Read the model definition and answer for the solid it produces. Units are mm, in the model's axes. Face numbers are marked on the shaded views. A direction names the side the tool comes from. Coordinates: 2 decimals unless noted, no trailing zeros. Loops run counter-clockwise (first coordinate to the right, second up) from the corner with the lowest first, then second, coordinate; pieces in that order, holes last. Notation, with made-up numbers: (-16.5, 14) -> (34.5, 14) arc R20 cw to (34.5, 41) -> close; hole circle Ø3 at (-28.75, 45). An arc over 180 degrees is marked (long way). Answer in a Markdown table with one row per item.
```python
from build123d import *
from build123d.topology import SkipClean

# Parameters (mm, degrees)
SKETCH1_R                    = 10.16
BOSS_EXTRUDE1_DEPTH          = 101.6
SKETCH3_R                    = 12.7
SKETCH3_R_2                  = 3.302
BOSS_EXTRUDE2_DEPTH          = 12.7
SKETCH5_W                    = 50.328091527
SKETCH5_H                    = 177.713548071
CUT_EXTRUDE2_DEPTH           = 122.062113097
SKETCH4_W                    = 0.976
SKETCH4_H                    = 5
CUT_EXTRUDE3_DEPTH           = 11.684
SKETCH4_3_R                  = 3.175
CUT_EXTRUDE4_DEPTH           = 6.35
CUT_EXTRUDE4_DRAFT           = -5
CUT_EXTRUDE4_PROFILE_2_DEPTH = 6.35
CUT_EXTRUDE4_PROFILE_2_DRAFT = -5
CUT_EXTRUDE4_PROFILE_3_DEPTH = 6.35
CUT_EXTRUDE4_PROFILE_3_DRAFT = -5
CUT_EXTRUDE4_PROFILE_4_DEPTH = 6.35
CUT_EXTRUDE4_PROFILE_4_DRAFT = -5
CUT_EXTRUDE5_DEPTH           = 124.013791019


with BuildPart() as part:
    # Sketch1 → Boss-Extrude1 (new body)
    with BuildSketch(Plane.XY):
        Circle(SKETCH1_R)
    extrude(amount=BOSS_EXTRUDE1_DEPTH)

    # Sketch2 → Revolve1 (revolve)
    with SkipClean():  # the faces are left unmerged after this step: merging them gives an invalid solid
        with BuildSketch(Plane(origin=(0, 0, 0), x_dir=(0, 0, -1), z_dir=(1, 0, 0))):
            with BuildLine():
                ThreePointArc((37.917636205, 0), (17.597636205, 20.32), (-2.722363795, 0))
                Line((-2.722363795, 0), (37.917636205, 0))
            make_face()
            with BuildLine():
                Line((37.917636205, 0), (-2.722363795, 0))
                ThreePointArc((-2.722363795, 0), (17.597636205, -20.32), (37.917636205, 0))
            make_face()
        revolve(axis=Axis((0, 0, 2.722363795), (0, 0, -1)))
    add(part.part.scale(1), mode=Mode.REPLACE)  # the faces are merged on a copy

    # Sketch3 → Boss-Extrude2 (add, symmetric)
    with BuildSketch(Plane(origin=(0, 0, 0), x_dir=(1, 0, 0), z_dir=(0, 1, 0))):
        with Locations(Location((0, -104.902, 0), (0, 0, 270))):
            Circle(SKETCH3_R)
        with Locations(Location((0, -104.902, 0), (0, 0, 270))):
            Circle(SKETCH3_R_2, mode=Mode.SUBTRACT)
    extrude(amount=BOSS_EXTRUDE2_DEPTH, both=True)

    # Sketch5 → Cut-Extrude2 (cut, through all)
    with BuildSketch(Plane(origin=(0, 0, 0), x_dir=(1, 0, 0), z_dir=(0, 1, 0))):
        with Locations((0.842814929, -41.287007492)):
            Rectangle(SKETCH5_W, SKETCH5_H)
    extrude(amount=CUT_EXTRUDE2_DEPTH, mode=Mode.SUBTRACT)

    # Sketch4 → Cut-Extrude3 (cut)
    with BuildSketch(Plane(origin=(0, 0, 0), x_dir=(1, 0, 0), z_dir=(0, 1, 0))):
        Polygon((-1.524, 11.040636205), (-1.524, 6.040636205), (1.524, 6.040636205), (1.524, 29.154636205), (-1.524, 29.154636205), (-1.524, 24.154636205), align=None)
        with Locations((-2.012, 8.540636205)):
            Rectangle(SKETCH4_W, SKETCH4_H)
        with Locations((-2.012, 26.654636205)):
            Rectangle(SKETCH4_W, SKETCH4_H)
    extrude(amount=-CUT_EXTRUDE3_DEPTH, mode=Mode.SUBTRACT)


with BuildPart() as cut_extrude4_tool:
    # Sketch4_3 → Cut-Extrude4 (with draft: the straight prism first)
    with BuildSketch(Plane(origin=(0, 0, 0), x_dir=(1, 0, 0), z_dir=(0, 1, 0))):
        with Locations((-11.43, 17.597636205)):
            Circle(SKETCH4_3_R)
    extrude(amount=-CUT_EXTRUDE4_DEPTH)
    # Cut-Extrude4: the draft: its side faces are tilted about the plane it starts from
    cut_extrude4_sides = [cut_extrude4_tool.faces().sort_by_distance(p)[0] for p in [
        (-14.605, -3.175, -17.597636205),
    ]]
    draft(cut_extrude4_sides, Plane(origin=(0, 0, 0), x_dir=(1, 0, 0), z_dir=(0, 1, 0)), CUT_EXTRUDE4_DRAFT)


with BuildPart() as part_1:
    add(part.part)

    # Cut-Extrude4: cut by cut_extrude4_tool
    add(cut_extrude4_tool.part, mode=Mode.SUBTRACT)


with BuildPart() as cut_extrude4_profile_2_tool:
    # Sketch4_3 → Cut-Extrude4 profile 2 (with draft: the straight prism first)
    with BuildSketch(Plane(origin=(0, 0, 0), x_dir=(1, 0, 0), z_dir=(0, 1, 0))):
        with Locations((11.43, 17.597636205)):
            Circle(SKETCH4_3_R)
    extrude(amount=-CUT_EXTRUDE4_PROFILE_2_DEPTH)
    # Cut-Extrude4 profile 2: the draft: its side faces are tilted about the plane it starts from
    cut_extrude4_profile_2_sides = [cut_extrude4_profile_2_tool.faces().sort_by_distance(p)[0] for p in [
        (8.255, -3.175, -17.597636205),
    ]]
    draft(cut_extrude4_profile_2_sides, Plane(origin=(0, 0, 0), x_dir=(1, 0, 0), z_dir=(0, 1, 0)), CUT_EXTRUDE4_PROFILE_2_DRAFT)


with BuildPart() as part_2:
    add(part_1.part)

    # Cut-Extrude4 profile 2: cut by cut_extrude4_profile_2_tool
    add(cut_extrude4_profile_2_tool.part, mode=Mode.SUBTRACT)


with BuildPart() as cut_extrude4_profile_3_tool:
    # Sketch4_3 → Cut-Extrude4 profile 3 (with draft: the straight prism first)
    with BuildSketch(Plane(origin=(0, 0, 0), x_dir=(1, 0, 0), z_dir=(0, 1, 0))):
        with Locations((0, -92.202)):
            Circle(SKETCH4_3_R)
    extrude(amount=-CUT_EXTRUDE4_PROFILE_3_DEPTH)
    # Cut-Extrude4 profile 3: the draft: its side faces are tilted about the plane it starts from
    cut_extrude4_profile_3_sides = [cut_extrude4_profile_3_tool.faces().sort_by_distance(p)[0] for p in [
        (-3.175, -3.175, 92.202),
    ]]
    draft(cut_extrude4_profile_3_sides, Plane(origin=(0, 0, 0), x_dir=(1, 0, 0), z_dir=(0, 1, 0)), CUT_EXTRUDE4_PROFILE_3_DRAFT)


with BuildPart() as part_3:
    add(part_2.part)

    # Cut-Extrude4 profile 3: cut by cut_extrude4_profile_3_tool
    add(cut_extrude4_profile_3_tool.part, mode=Mode.SUBTRACT)


with BuildPart() as cut_extrude4_profile_4_tool:
    # Sketch4_3 → Cut-Extrude4 profile 4 (with draft: the straight prism first)
    with BuildSketch(Plane(origin=(0, 0, 0), x_dir=(1, 0, 0), z_dir=(0, 1, 0))):
        with BuildLine():
            Line((-10.16, -87.162), (-10.16, -92.162))
            ThreePointArc((-10.16, -92.162), (-1.20802815, -88.45397185), (2.5, -79.502))
            Line((2.5, -79.502), (2.5, 6.040636205))
            Line((2.5, 6.040636205), (-2.5, 6.040636205))
            Line((-2.5, 6.040636205), (-2.5, -79.502))
            ThreePointArc((-2.5, -79.502), (-4.743562056, -84.918437944), (-10.16, -87.162))
        make_face()
    extrude(amount=-CUT_EXTRUDE4_PROFILE_4_DEPTH)
    # Cut-Extrude4 profile 4: the draft: its side faces are tilted about the plane it starts from
    cut_extrude4_profile_4_sides = [cut_extrude4_profile_4_tool.faces().sort_by_distance(p)[0] for p in [
        (-4.743562056, -3.175, 84.918437944),
        (-10.16, -3.175, 89.662),
        (-1.20802815, -3.175, 88.45397185),
        (2.5, -3.175, 36.730681898),
        (0, -3.175, -6.040636205),
        (-2.5, -3.175, 36.730681898),
    ]]
    draft(cut_extrude4_profile_4_sides, Plane(origin=(0, 0, 0), x_dir=(1, 0, 0), z_dir=(0, 1, 0)), CUT_EXTRUDE4_PROFILE_4_DRAFT)


with BuildPart() as part_4:
    add(part_3.part)

    # Cut-Extrude4 profile 4: cut by cut_extrude4_profile_4_tool
    add(cut_extrude4_profile_4_tool.part, mode=Mode.SUBTRACT)

    # Sketch7 → Cut-Extrude5 (cut, through all)
    with BuildSketch(Plane(origin=(-10.082823385, -0.882132743, 0), x_dir=(0, 0, -1), z_dir=(0.9961946980917457, 0.08715574274765837, 1.0368733976540235e-15))):
        Polygon((-92.006694168, -0.885502346), (-92.162, 0.885502346), (-87.162, 0.885502346), (-87.314828647, -0.885502346), align=None)
    extrude(amount=-CUT_EXTRUDE5_DEPTH, mode=Mode.SUBTRACT)


solid = part_4.part
```
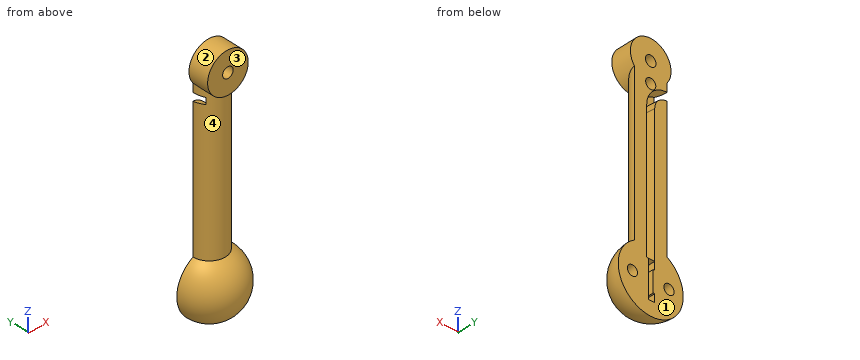
1. A cutting plane is placed at D-D on z = -2. Give the vertices of the cut face in (x, y), and give its area (3 significant figures).
A:
| item | result |
|---|---|
| outline | (-13.02, 0) arc R13.02 ccw to (13.02, 0) -> (2.5, 0) -> (1.94, -6.35) -> (-1.94, -6.35) -> (-2.5, 0) -> close |
| area | 238 mm2 |
2. The mould has two halves that part along Z. Classify the marked faces 1 and 2: pulls with the +Z half, pulls with the -Z half, needs draft (parallel to the pull), parting line crosses it, or undercut.
A:
| item | result |
|---|---|
| face 1 | needs draft |
| face 2 | undercut |
3. A cutting plane is placed at A-A on z = 75.5. Give the vertices of the cut face in (x, y), and give its area (3 significant figures).
A:
| item | result |
|---|---|
| outline | (-10.16, 0) arc R10.16 ccw to (10.16, 0) -> (2.5, 0) -> (1.94, -6.35) -> (-1.94, -6.35) -> (-2.5, 0) -> close |
| area | 134 mm2 |
4. A tool of negligible diameter and unlimited length cuts with its end or side. For the marked faces 3 and 4, from which of +Z, -Z, +X, -X, +Y, -Y can it reach the whole face along a straight path? Write none if from no direction.
A:
| item | result |
|---|---|
| face 3 | +Z, +X, -X, -Y |
| face 4 | -Y |
5. Find the intervals of material crossed by probe 1 along Z at (x, y) = (0, -3.25); probe 2 along Z at (x, y) = (0, -10); probe 3 along Z at (x, y) = (0, -8.5), in increasing order.
A:
| item | result |
|---|---|
| probe 1 | z = -37.66 to -29.15, -6.04 to -5.76, 86.57 to 89.31, 95.09 to 101.6, 108.2 to 117.6 |
| probe 2 | z = -35.29 to -29.15, -6.04 to 101.6, 108.2 to 117.6 |
| probe 3 | z = -36.05 to -29.15, -6.04 to 101.6, 108.2 to 117.6 |
6. Given pin 1 Ø1.2 at (x, z) = (-0.5, -13) entering from +Y; pin 2 Ø5 at (x, z) = (-6.5, 26.5) entering from -Y; pin 3 Ø10 at (x, z) = (-16, 15.5) entering from -Y; pin 4 Ø6 at (x, y) = (1.5, -13.5) entering from -Z, each flat-ended and moving along its own axis, determine where each tip first touches the part or whether it passes through.
A:
| item | result |
|---|---|
| pin 1 | stops at y = -11.68 |
| pin 2 | stops at y = -9.34 |
| pin 3 | passes through |
| pin 4 | stops at z = -34.94 |
7. A cutting plane is placed at B-B on y = -18.5. Give the vertices of the cut face in (x, z).
A:
| item | result |
|---|---|
| outline | circle Ø16.81 at (0, -17.6) |
